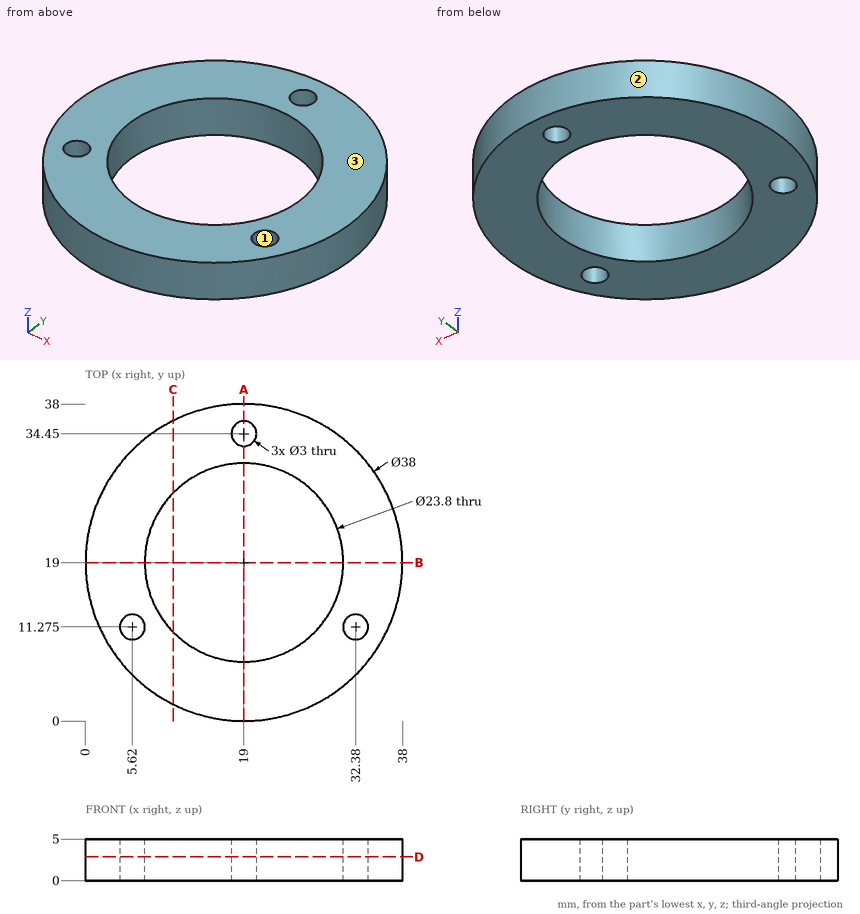
Answer from the drawing. Dimensions are ordinates in mm from the lowest x, y and z of the part. Give positions to 0.01 mm unless a question says otherwise; leave off trailing zeros. Loops run counter-clockwise (first coordinate to the right, second up) from the corner with the lowest first, then second, coordinate; pieces in that order, holes last.
Item 1: A cutting plane is placed at B-B (y = 19). Give the vertices of the cut face in (x, z).
Derived:
outline: (0, 0) - (7.1, 0) - (7.1, 5) - (0, 5) - close; (30.9, 0) - (38, 0) - (38, 5) - (30.9, 5) - close
Item 2: A cutting plane is placed at C-C (x = 10.5). Give the vertices of the cut face in (y, z).
Derived:
outline: (2.01, 0) - (10.67, 0) - (10.67, 5) - (2.01, 5) - close; (27.33, 0) - (35.99, 0) - (35.99, 5) - (27.33, 5) - close
Item 3: Each of these flat-tipped pins is pushed along its axis until it touches: pin 1 Ø5 at (x, y) = (12, 22.5) entering from -Z (3 decimals); pin 2 Ø3 at (x, z) = (15, 4.5) entering from +Y; pin 3 Ø2 at (x, z) = (27, 2) entering from -Y; pin 4 Ø2 at (x, z) = (20, 3.5) entering from -Y. Where does it stop, or does it pass through?
Derived:
pin 1: passes through
pin 2: stops at y = 37.83
pin 3: stops at y = 1.34
pin 4: stops at y = 0
Item 4: A cutting plane is placed at A-A (x = 19). Give the vertices of the cut face in (y, z).
Derived:
outline: (0, 0) - (7.1, 0) - (7.1, 5) - (0, 5) - close; (30.9, 0) - (32.95, 0) - (32.95, 5) - (30.9, 5) - close; (35.95, 0) - (38, 0) - (38, 5) - (35.95, 5) - close
Item 5: A cutting plane is placed at D-D (z = 2.85). Give the vertices of the cut face in (x, y) (3 decimals), then the cut area to 3 significant figures.
Derived:
outline: circle Ø38 at (19, 19); hole circle Ø3 at (5.62, 11.275); hole circle Ø23.8 at (19, 19); hole circle Ø3 at (19, 34.45); hole circle Ø3 at (32.38, 11.275)
area: 668 mm2
Item 6: Find the intervals of material crossed by line 1 along Y through (x, z) = (19, 2.25); line 2 along Y through (x, z) = (12, 1); line 3 along X through (y, z) = (21, 4.7), in increasing order.
Derived:
line 1: y = 0 to 7.1, 30.9 to 32.95, 35.95 to 38
line 2: y = 1.34 to 9.38, 28.62 to 36.66
line 3: x = 0.11 to 7.27, 30.73 to 37.89
Item 7: Determine the mould class of the marked faces 1, 2 and 3 for opening direction X: +X half, -X half, draft (parallel to the pull), parting line (faces both ways), or undercut.
Derived:
face 1: undercut
face 2: parting line
face 3: draft
